Input: part model. Units: mm. Frame: model coordinates. A direction names the side the tool comes from. Coordinates: 2 decimals unless noted, no trailing zeros. Write each loop counter-clockwise with the first axis right and the second up, starting at its lowest first coordinate (ties: lowest second). Pieces come first, ordered by that corner, then holes.
Autodesk Inventor part; units mm, degrees
ref_plane "Arbeitsebene2" through (31.75, -29, 35) normal (0, 0, 1) x (1, 0, 0)
ref_plane "YZ Plane" through (0, 0, 0) normal (1, 0, 0) x (0, 1, 0)
ref_plane "XZ Plane" through (0, 0, 0) normal (0, 1, 0) x (-1, 0, 0)
ref_plane "Arbeitsebene1" through (0, 0, 0) normal (0, 0, 1) x (1, 0, 0)
sketch "Skizze1" plane through (0, 0, 0) normal (0, 0, 1) x (1, 0, 0)
  circle A0 centre (-1.9028, 0) radius 18.75
  circle A1 centre (-1.9028, 0) radius 16.25
  line L0 (31.75, -9) -> (39.5, -9)
  line L1 (39.5, -9) -> (39.5, -29)
  circle A2 centre (-1.9028, 0) radius 17.0624
  line L2 (39.9814, -7.7741) -> (15.1596, -7.7741)
  line L3 (15.1596, -7.7741) -> (15.1596, 0)
  line L4 (15.1596, 0) -> (39.9814, 0)
  line L5 (39.9814, 0) -> (39.9814, -7.7741)
  line L6 (39.9814, 0) -> (42.9814, 0)
  line L7 (42.9814, 0) -> (42.9814, -28.4525)
  line L8 (42.9814, -28.4525) -> (39.9814, -28.4525)
  line L9 (39.9814, -28.4525) -> (39.9814, 0)
  point P0 (0, 0)
  dimension "d0" = 3
extrude "Extrusion1" add sketch "Skizze1" along normal blind 5 contours L4 L3 A0 | L4 L5 L2 A0 | A0 L3 L4 | L6 L7 L8 L9 L5
sketch "Skizze2" plane through (0, 0, 5) normal (0, 0, 1) x (1, 0, 0)
  arc A0 (16.8472, 0) -> (15.1596, -7.7741) centre (-1.9028, 0) ccw
  line L0 (15.1596, -7.7741) -> (39.9814, -7.7741)
  line L1 (39.9814, -7.7741) -> (39.9814, -28.4525)
  line L2 (39.9814, -28.4525) -> (42.9814, -28.4525)
  line L3 (42.9814, -28.4525) -> (42.9814, 0)
  line L4 (42.9814, 0) -> (16.8472, 0)
  circle A1 centre (-1.9028, 0) radius 17.0624
  line L5 (42.9814, 0) -> (39.9814, 0)
  line L6 (39.9814, 0) -> (39.9814, -28.4525)
  line L7 (39.9814, -28.4525) -> (42.9814, -28.4525)
  line L8 (42.9814, -28.4525) -> (42.9814, 0)
  point P0 (0, 0)
ref_plane "Arbeitsebene2" through (31.75, -29, 35) normal (0, 0, 1) x (1, 0, 0)
extrude "Extrusion2" add sketch "Skizze2" along normal up to surface (30 mm away) contours L4 L3 L2 L1 L6
sketch "Skizze3" plane through (42.9814, -28.4525, 0) normal (1, 0, 0) x (0, 0, -1)
  line L0 (-35, 13.9525) -> (6, 13.9525)
  line L1 (-35, 13.9525) -> (6, 13.9525)
  circle A0 centre (-6, 16.9525) radius 1.5
  circle A1 centre (-23, 16.9525) radius 1.5
  circle A2 centre (-6, 2.2025) radius 1.5
  circle A3 centre (-23, 1.9525) radius 1.5
  circle A4 centre (-23, 25.4997) radius 1.5
  circle A5 centre (-7.5, 25.4997) radius 1.5
  point P0 (0, 28.4525)
  dimension "d7" = 3
  dimension "d8" = 3
extrude "Extrusion3" cut sketch "Skizze3" against normal blind 5
properties part number "16_Gabel"
Item 1: Access query for faces 4 (the face through (28, -7.774, 2)), 5 (the face through (35, 0, 3)), 6 (the face through (41.5, -12.4, 7.2)). Directions: +Z, -Z, +X, -X, +Y, -Y. A direction counts if a zero-diameter tool reaches every point of the face in a straight line with its end or side. Return the directions, or none.
Item 2: Section query C-C, the plane z = 19.5. Return loops of the section in (x, y).
Item 3: Pull-direction query (Z, two-part tool) for faces 1 (the face through (41, -14, 35)), 2 (the face through (41.5, -11.43, 24.5)), 3 (the face through (16, -3, 0)); classes: released by +Z, released by -Z, zero draft, split by the parting line, or undercut.
Item 4: Section query D-D, the plane y = -19.5. Return loops of the section in (x, z), then the cut area to 3 significant figures.
Item 5: Section query B-B, the plane y = 12. Return loops of the section in (x, z), then the cut area to 3 significant figures.
Item 6: Section query A-A, the plane z = 23. Return loops of the section in (x, y).
Item 7: Material intervals for line 1 (Y direction, x = 42.3, z = 23); line 2 (X direction, y = -10, z = 19); line 3 (Z direction, x = 13, y = -9), sorted ascending.
Item 8: Pin query (flat end, axial travel): pin 1 Ø21 at (x, z) = (34.5, 17) entering from +Y; pin 2 Ø10 at (x, z) = (8, 4.5) entering from -Y; pin 3 Ø2.5 at (y, z) = (-2.95, 23) entering from +X; pin 4 Ø14 at (y, z) = (-20, 20.5) entering from -X. Return the tip coordinate at first contact, or that it passes through.
The answers:
1. face 4: +Z, -Z, -Y
1. face 5: +Z, -Z, +X, +Y
1. face 6: +X
2. outline: (39.98, -28.45) - (42.98, -28.45) - (42.98, 0) - (39.98, 0) - close
3. face 1: released by +Z
3. face 2: undercut
3. face 3: released by -Z
4. outline: (39.98, 0) - (42.98, 0) - (42.98, 35) - (39.98, 35) - close
4. area: 105 mm2
5. outline: (-16.31, 0) - (-14.03, 0) - (-14.03, 5) - (-16.31, 5) - close; (10.23, 0) - (12.5, 0) - (12.5, 5) - (10.23, 5) - close
5. area: 22.8 mm2
6. outline: (39.98, -28.45) - (42.98, -28.45) - (42.98, -28) - (39.98, -28) - close; (39.98, -25) - (42.98, -25) - (42.98, -13) - (39.98, -13) - close; (39.98, -10) - (42.98, -10) - (42.98, -4.45) - (39.98, -4.45) - close; (39.98, -1.45) - (42.98, -1.45) - (42.98, 0) - (39.98, 0) - close
7. line 1: y = -28.45 to -28, -25 to -13, -10 to -4.45, -1.45 to 0
7. line 2: x = 39.98 to 42.98
7. line 3: z = 0 to 5
8. pin 1: stops at y = 0
8. pin 2: stops at y = -18.1
8. pin 3: passes through
8. pin 4: stops at x = 39.98
